```python
from build123d import *

# Parameters (mm, degrees)
SKETCH1_W           = 60
SKETCH1_H           = 18
BOSS_EXTRUDE1_DEPTH = 75
SKETCH2_W           = 18
SKETCH2_H           = 65
CUT_EXTRUDE1_DEPTH  = 15
FILLET1_SIZE        = 10
FILLET1_SIZE_2      = 2


with BuildPart() as part:
    # Sketch1 → Boss-Extrude1 (new body)
    with BuildSketch(Plane(origin=(0, 0, 0), x_dir=(1, 0, 0), z_dir=(0, 1, 0))):
        with Locations((0, -9)):
            Rectangle(SKETCH1_W, SKETCH1_H)
    extrude(amount=BOSS_EXTRUDE1_DEPTH)

    # Sketch2 → Cut-Extrude1 (cut)
    with BuildSketch(Plane.XY.offset(18)):
        with Locations((-19.5, 37.5)):
            Rectangle(SKETCH2_W, SKETCH2_H)
        with Locations((0, 37.5)):
            Rectangle(SKETCH2_W, SKETCH2_H)
        with Locations((19.5, 37.5)):
            Rectangle(SKETCH2_W, SKETCH2_H)
    extrude(amount=-CUT_EXTRUDE1_DEPTH, mode=Mode.SUBTRACT)

    # Fillet1
    # an asymmetric fillet: 10, 2 mm, written as the material it takes off along each edge
    with BuildSketch(Plane(origin=(-30, -25, 18), x_dir=(0, 0, -1), z_dir=(0, 1, 0))) as fillet1_piece_1:
        with BuildLine():
            Bezier((FILLET1_SIZE, 0), (0, 0), (0, -FILLET1_SIZE_2), weights=[1, 0.707106781, 1])
            Line((0, -FILLET1_SIZE_2), (0, 0))
            Line((0, 0), (FILLET1_SIZE, 0))
        make_face()
    extrude(amount=125, mode=Mode.SUBTRACT)
    with BuildSketch(Plane(origin=(30, -25, 18), x_dir=(0, 0, -1), z_dir=(0, 1, 0))) as fillet1_piece_2:
        with BuildLine():
            Bezier((FILLET1_SIZE, 0), (0, 0), (0, FILLET1_SIZE_2), weights=[1, 0.707106781, 1])
            Line((0, FILLET1_SIZE_2), (0, 0))
            Line((0, 0), (FILLET1_SIZE, 0))
        make_face()
    extrude(amount=125, mode=Mode.SUBTRACT)


solid = part.part
```
Part model, mm, in its own coordinate system. A direction names the side the tool comes from. Coordinates: 2 decimals unless noted, no trailing zeros. Order: outer loops, then holes, each group sorted by start corner. A loop starts at its lowest first (then second) coordinate and runs counter-clockwise, first axis right, second up. Notation, with made-up numbers: (74.25, 9.5) -> (131.25, 9.5) arc R24 ccw to (131.25, 33.5) -> close; hole circle Ø5 at (27, 86.25). An arc over 180 degrees is marked (long way). Put each result on its own line as item: value. Start each with the question number.
(1) Band-saw the part on C-C (z = 14). Count the separate pieces of the cut face and the enclosed holes in it, then the cut area to 3 significant figures.
(2) Band-saw the part on A-A (z = 5.5). Give the cut face in (x, y).
(3) Which spindle directions (+Z, -Z, +X, -X, +Y, -Y) get a long thin tool onto all of the face, cutting with end or side? Do faces 4 (the face through (-20, 5, 11)), 5 (the face through (30, 37, 4)). Say none if no direction does.
(4) Band-saw the part on B-B (x = -13.5). Give the cut face in (y, z), then the cut area to 3 significant figures.
(5) Probe line 1 along X through (y, z) = (69.5, 5.5); line 2 along Y through (x, z) = (15, 14.75); line 3 along X through (y, z) = (12, 13.25). List the from-to ranges inside material, lowest first. Write a range as [from, to].
(6) Pin check, flat tips, straight feed: pin 1 Ø4.5 at (y, z) = (26, 13.5) entering from +X; pin 2 Ø8 at (x, y) = (16, 61) entering from +Z. Stop position of each tip, or through.
(7) Mould opens along Y. For faces 1 (the face through (-9, 37, 11)), 2 (the face through (0, 75, 9)), 3 (the face through (0, 37, 0)) say: pulls with the +Y half, pulls with the -Y half, needs draft (parallel to the pull), parting line crosses it, or undercut.
Determined:
1. separate pieces: 1
1. enclosed holes: 3
1. area: 930 mm²
2. outline: (-30, 0) -> (30, 0) -> (30, 75) -> (-30, 75) -> close; hole (-28.5, 5) -> (-10.5, 5) -> (-10.5, 70) -> (-28.5, 70) -> close; hole (-9, 5) -> (9, 5) -> (9, 70) -> (-9, 70) -> close; hole (10.5, 5) -> (28.5, 5) -> (28.5, 70) -> (10.5, 70) -> close
3. face 4: +Z
3. face 5: +Z, -Z, +X, +Y, -Y
4. outline: (0, 0) -> (75, 0) -> (75, 18) -> (70, 18) -> (70, 3) -> (5, 3) -> (5, 18) -> (0, 18) -> close
4. area: 375 mm²
5. line 1: x = [-30, -28.5], [-10.5, -9], [9, 10.5], [28.5, 30]
5. line 2: y = [0, 5], [70, 75]
5. line 3: x = [-29.7, -28.5], [-10.5, -9], [9, 10.5], [28.5, 29.7]
6. pin 1: stops at x = 29.89
6. pin 2: stops at z = 3
7. face 1: undercut
7. face 2: pulls with the +Y half
7. face 3: needs draft
